Can you work these out from the model? Positions are in its coordinate system, mm. A direction names the side the tool comes from. Give positions to 0.01 mm unless a question says otherwise; leave off trailing zeros. Loops run counter-clockwise (first coordinate to the right, second up) from the corner with the lowest first, then second, coordinate; pieces in that order, holes last. Notation, with made-up numbers: M 29,-39.5 L 72,-39.5 A17 cw 72,-31.5 Z; hole C -33,7.5 d2. An arc over 180 degrees is marked long. Use CSV: the item, a comma, the result in double quotes.
from build123d import *

# Parameters (mm, degrees)
F2_R = 25.4
F3_R = 5.08


with BuildPart() as f1:
    # F0 (on Front) → F1 (revolve)
    with BuildSketch(Plane.XZ):
        Polygon((22.225, 228.6), (19.05, 228.6), (19.05, 202.88843), (47.625, 182.88), (47.625, 3.175), (0, 3.175), (0, 0), (47.625, 0), (50.8, 0), (50.8, 187.96), (22.225, 207.96843), align=None)
    revolve(axis=Axis((0, 0, 114.3), (0, 0, 1)))

    # F2
    f2_edges = [f1.edges().sort_by_distance(p)[0] for p in [
        (-50.8, 0, 187.96),
    ]]
    fillet(f2_edges, radius=F2_R)

    # F3
    f3_edges = [f1.edges().sort_by_distance(p)[0] for p in [
        (-50.8, 0, 0),
    ]]
    fillet(f3_edges, radius=F3_R)


solid = f1.part
Q1. If we mould it in two halves opening along X, with no side actions, what happens to faces 3 (the cylindrical face through (-15.12, -11.59, 215.56)), 4 (the flat face through (16.4, 10, 228.6)), 5 (the cylindrical face through (21.199, 6.676, 218.429))? For each: released by +X, released by -X, zero draft, split by the parting line, or undercut.
Model answer:
face 3,"undercut"
face 4,"zero draft"
face 5,"split by the parting line"
Q2. For faces 1 (the cylindrical face through (27.31, 42.835, 91.096)), 2 (the flat face through (-1, 1, 3.175)), which set-ups out of +Z, -Z, +X, -X, +Y, -Y let a thin tool reach every point of the face, with its end or its side?
Model answer:
face 1,"+Z, -Z"
face 2,"none"
Q3. I want a section at A-A, the plane z = 212.5. Please give me the cut outline in (x, y) (3 decimals), then the cut area to 3 significant figures.
Model answer:
outline,"C 0,0 d44.45; hole C 0,0 d38.1"
area,"412 mm2"
Q4. I want a section at B-B, the plane z = 121. Please give me the cut outline in (x, y) (3 decimals).
Model answer:
outline,"C 0,0 d101.6; hole C 0,0 d95.25"
Q5. I'm going to push flat-ended pins straight in: P1, Ø2, axis at x = 8, z = 57, coming from the +Y side; P2, Ø4, axis at y = -30, z = 81.5, coming from the +X side; P3, Ø1, axis at y = 17.5, z = 63, coming from the -X side. Where does each tip first touch, or does it pass through?
Model answer:
P1,"y = 50.32"
P2,"x = 42.39"
P3,"x = -47.87"
Q6. Please list where these lines run through material, in increasing order: L1, parallel to Y at x = 0, z = 45.5 (3 decimals); L2, parallel to Y at x = 0, z = 220 (3 decimals); L3, parallel to Z at x = 3.5, y = 21.5 (3 decimals). Write a range as from..to.
Model answer:
L1,"-50.8..-47.625, 47.625..50.8"
L2,"-22.225..-19.05, 19.05..22.225"
L3,"0..3.175, 200.975..228.6"
